from build123d import *

# Parameters (mm, degrees)
F1_DEPTH  = 25.4
F2_W      = 43.18
F2_H      = 45.72
F2_W_2    = 39.116
F2_H_2    = 41.656
F3_DEPTH  = 10.16
F4_W      = 43.18
F4_H      = 45.72
F5_DEPTH  = 2.54
F6_W      = 39.116
F6_H      = 3.175
F7_DEPTH  = 25.4
F9_DEPTH  = 3.175
F11_DEPTH = 3.175


with BuildPart() as f1:
    # F0 (on Front) → F1 (new body)
    with BuildSketch(Plane.XZ):
        Polygon((0, 34.925), (0, 0), (81.28, 0), (81.28, 34.925), (60.98439, 34.925), (60.98439, 31.75), (78.105, 31.75), (78.105, 3.175), (3.175, 3.175), (3.175, 31.75), (15.319279, 31.75), (15.319279, 34.925), align=None)
    extrude(amount=F1_DEPTH)

    # F2 (on face) → F3 (join)
    with BuildSketch(Plane(origin=(0, 0, 0), x_dir=(1, 0, 0), z_dir=(0, 0, -1))):
        with Locations((40.64, 12.7)):
            Rectangle(F2_W, F2_H)
        with Locations((40.64, 12.7)):
            Rectangle(F2_W_2, F2_H_2, mode=Mode.SUBTRACT)
    extrude(amount=F3_DEPTH)

    # F4 (on face) → F5 (join)
    with BuildSketch(Plane(origin=(0, 0, -10.16), x_dir=(1, 0, 0), z_dir=(0, 0, -1))):
        with Locations((40.64, 12.7)):
            Rectangle(F4_W, F4_H)
    extrude(amount=F5_DEPTH)

    # F6 (on face) → F7 (cut)
    with BuildSketch(Plane(origin=(0, 0, 0), x_dir=(-1, 0, 0), z_dir=(0, 1, 0))):
        with Locations((-40.64, 1.5875)):
            Rectangle(F6_W, F6_H)
    extrude(amount=-F7_DEPTH, mode=Mode.SUBTRACT)

    # F8 (on face) → F9 (join)
    with BuildSketch(Plane.XY):
        Polygon((19.05, 10.16), (19.05, 0), (21.082, 0), (21.082, 8.128), (60.198, 8.128), (60.198, 0), (62.23, 0), (62.23, 10.16), align=None)
    extrude(amount=F9_DEPTH)

    # F10 (on face) → F11 (join)
    with BuildSketch(Plane.XY):
        Polygon((21.082, -25.4), (19.05, -25.4), (19.05, -35.56), (62.23, -35.56), (62.23, -25.4), (60.198, -25.4), (60.198, -33.528), (21.082, -33.528), align=None)
    extrude(amount=F11_DEPTH)


solid = f1.part
CAD build for the part. Positions are in the model's coordinates, mm. A direction names the side the tool comes from. Coordinates: 2 decimals unless noted, no trailing zeros. Write each loop counter-clockwise with the first axis right and the second up, starting at its lowest first coordinate (ties: lowest second). Pieces come first, ordered by that corner, then holes. Notation, with made-up numbers: M 27.5,32.5 L 41.5,32.5 A14 cw 41.5,47.5 Z; hole C 22,46.25 d4. An arc over 180 degrees is marked long. Answer as a JSON object with one key per item and string values. Group by question number.
1) Tool access for faces 1 (the face through (40, -13, -10.16)), 2 (the face through (71, -13, 34.925)), 3 (the face through (9, -13, 31.75)), 4 (the face through (60.984, -13, 33)), 5 (the face through (9, -13, 0)): list every direction of +Z, -Z, +X, -X, +Y, -Y with a clear straight run to the whole face (end or side of a thin tool).
2) Saw through at B-B (y = -2). Write the cut outline in (x, z) (3 decimals).
3) Saw through at A-A (z = 4.5). Write the cut outline in (x, y) (3 decimals).
4) Wall check: line 1 (Y direction, x = 50, z = -6); line 2 (Z direction, x = 76, y = -4.5) (3 decimals); line 3 (X direction, y = 7, z = 3). Give the ranges that are in metal, low to high. Write a range as from..to.
5) Mould opens along X. For faces 6 (the face through (0, -13, 18)), 7 (the face through (78.105, -13, 18)), 8 (the face through (8, -13, 34.925)) say: +X half, -X half, draft (parallel to the pull), parting line (faces both ways), or undercut.
6) Saw through at C-C (z = -5). Write the cut outline in (x, y).
7) Saw through at D-D (x = 30.5). Write the cut outline in (y, z) (3 decimals), plus the area to 3 significant figures.
8) Pin check, flat tips, straight feed: pin 1 Ø21 at (x, z) = (9, 16) entering from -Y; pin 2 Ø13.5 at (x, y) = (12, -16.5) entering from -Z; pin 3 Ø15 at (x, z) = (7.5, 19) entering from +Y. Stop position of each tip, or through.
Values follow:
{
 "1": {"face 1": "+Z", "face 2": "+Z, +X, -X, +Y, -Y", "face 3": "+Y, -Y", "face 4": "+Z, +Y, -Y", "face 5": "-Z, -X, +Y, -Y"},
 "2": {"outline": "M 0,0 L 19.05,0 L 19.05,-12.7 L 62.23,-12.7 L 62.23,0 L 81.28,0 L 81.28,34.925 L 60.984,34.925 L 60.984,31.75 L 78.105,31.75 L 78.105,3.175 L 60.198,3.175 L 60.198,-10.16 L 21.082,-10.16 L 21.082,3.175 L 3.175,3.175 L 3.175,31.75 L 15.319,31.75 L 15.319,34.925 L 0,34.925 Z"},
 "3": {"outline": "M 0,-25.4 L 3.175,-25.4 L 3.175,0 L 0,0 Z; M 78.105,-25.4 L 81.28,-25.4 L 81.28,0 L 78.105,0 Z"},
 "4": {"line 1": "y = -35.56..-33.53, 8.13..10.16", "line 2": "z = 0..3.175, 31.75..34.925", "line 3": "x = 19.05..21.08, 60.2..62.23"},
 "5": {"face 6": "-X half", "face 7": "undercut", "face 8": "draft"},
 "6": {"outline": "M 19.05,-35.56 L 62.23,-35.56 L 62.23,10.16 L 19.05,10.16 Z; hole M 21.08,-33.53 L 60.2,-33.53 L 60.2,8.13 L 21.08,8.13 Z"},
 "7": {"outline": "M -35.56,-12.7 L 10.16,-12.7 L 10.16,3.175 L 8.128,3.175 L 8.128,-10.16 L -33.528,-10.16 L -33.528,3.175 L -35.56,3.175 Z", "area": "170 mm2"},
 "8": {"pin 1": "stops at y = -25.4", "pin 2": "stops at z = 0", "pin 3": "stops at y = 0"}
}
